For this review, take the finished solid that the model builds, in its own axes (mm). A direction names the side the tool comes from. Round coordinates to 2 decimals unless told otherwise and drop trailing zeros. Loops run counter-clockwise (first coordinate to the right, second up) from the corner with the lowest first, then second, coordinate; pieces in that order, holes last. Notation, with made-up numbers: (-31, -15.75) -> (-13, -15.75) arc R35 ccw to (-13, 16.25) -> close; hole circle Ø2 at (57, 31). An arc over 180 degrees is marked (long way). Write each question's results on one line, items separated by ' | '.
```python
from build123d import *

# Parameters (mm, degrees)
SKETCH2_W               = 300
SKETCH2_H               = 292.795139568
SKETCH2_H_2             = 222.204860432
SKETCH2_H_3             = 20
BOSS_EXTRUDE1_DEPTH     = 20
SHELL1_T                = -1
SKETCH3_W               = 2
SKETCH3_H               = 20
BOSS_EXTRUDE2_DEPTH     = 40
CUT_EXTRUDE1_DEPTH      = 960.966652524
CUT_EXTRUDE1_DEPTH_BACK = 960.966652524
SKETCH4_R               = 3.5
CUT_EXTRUDE2_DEPTH      = 847.070903624
CUT_EXTRUDE2_DEPTH_BACK = 847.070903624
SKETCH5_R               = 3.5


with BuildPart() as part:
    # Sketch2 → Boss-Extrude1 (new body)
    with BuildSketch(Plane.XY):
        Polygon((-19.075846715, -602.110166283), (-189.075846715, -602.110166283), (-189.075846715, -627.110166283), (500.924153285, -627.110166283), (500.924153285, -602.110166283), (330.924153285, -602.110166283), (330.924153285, -2.110166283), (-19.075846715, -2.110166283), align=None)
        with Locations((155.924153285, -173.507736067)):
            Rectangle(SKETCH2_W, SKETCH2_H, mode=Mode.SUBTRACT)
        with Locations((155.924153285, -491.007736067)):
            Rectangle(SKETCH2_W, SKETCH2_H_2, mode=Mode.SUBTRACT)
        with Locations((155.924153285, -349.905305851)):
            Rectangle(SKETCH2_W, SKETCH2_H_3, mode=Mode.SUBTRACT)
    extrude(amount=BOSS_EXTRUDE1_DEPTH)

    # Shell1
    shell1_openings = [part.faces().sort_by_distance(p)[0] for p in [
        (500.924153285, -614.610166283, 10),
        (-189.075846715, -614.610166283, 10),
    ]]
    offset(amount=SHELL1_T, openings=shell1_openings, kind=Kind.INTERSECTION)

    # Sketch3 → Boss-Extrude2 (add)
    with BuildSketch(Plane.XZ.offset(627.110166283)):
        with Locations((493.924153285, 10)):
            Rectangle(SKETCH3_W, SKETCH3_H)
        with Locations((-182.075846715, 10)):
            Rectangle(SKETCH3_W, SKETCH3_H)
    extrude(amount=BOSS_EXTRUDE2_DEPTH)

    # Sketch4 → Cut-Extrude1 (cut, two sides: drawn at the far end of the back side and taken through both)
    with BuildSketch(Plane.ZY.offset(189.075846715).offset(-CUT_EXTRUDE1_DEPTH_BACK)):
        with Locations((10, -652.110166283)):
            Circle(SKETCH4_R)
    extrude(amount=CUT_EXTRUDE1_DEPTH + CUT_EXTRUDE1_DEPTH_BACK, mode=Mode.SUBTRACT)

    # Sketch5 → Cut-Extrude2 (cut, two sides: drawn at the far end of the back side and taken through both)
    with BuildSketch(Plane.ZY.offset(19.075846715).offset(-CUT_EXTRUDE2_DEPTH_BACK)):
        with Locations(Location((10, -273.200166283, 0), (0, 0, 270))):
            Circle(SKETCH5_R)
    extrude(amount=CUT_EXTRUDE2_DEPTH + CUT_EXTRUDE2_DEPTH_BACK, mode=Mode.SUBTRACT)


solid = part.part
```
1. Consider section A-A (x = 177.5). Give the number of separate pieces and of enclosed holes in the cut face, plus the area to 3 significant figures.
Values found:
separate pieces: 4 | enclosed holes: 4 | area: 324 mm2
2. Consider section C-C (y = -613.5). State the section outline as (x, z) points, plus the area to 3 significant figures.
Values found:
outline: (-189.08, 0) -> (500.92, 0) -> (500.92, 1) -> (-189.08, 1) -> close; (-189.08, 19) -> (500.92, 19) -> (500.92, 20) -> (-189.08, 20) -> close | area: 1,380 mm2
3. Tool access review of faces 4 (the face through (154, -602.11, 10)), 5 (the face through (492.924, -647, 10)), 6 (the face through (306.924, -176, 10)): name each direction out of +Z, -Z, +X, -X, +Y, -Y from which nothing blocks a thin tool from reaching the whole face with its end or side.
Values found:
face 4: +Z, -Z | face 5: +Z, -Z, -Y | face 6: none
4. To check wall thickness, follow probe 1 along X at (y, z) = (-52, 7); probe 2 along Y at (x, z) = (494.3, 10); probe 3 along Y at (x, z) = (5.5, 9.75). State the ranges of each line that lie inside material, in increasing order.
Values found:
probe 1: x = -19.08 to -18.08, 4.92 to 5.92, 305.92 to 306.92, 329.92 to 330.92 | probe 2: y = -667.11 to -655.61, -648.61 to -626.11, -603.11 to -602.11 | probe 3: y = -627.11 to -626.11, -603.11 to -378.91, -360.91 to -338.91, -320.91 to -276.69, -269.71 to -26.11, -3.11 to -2.11
5. For pin 1 (3 mm diameter, centred on x = -185.5, z = 7.5, fed in from -Y); pin 2 (5 mm diameter, centred on x = 365.5, z = 7.5, fed in from +Y); pin 3 (11 mm diameter, centred on y = -652.11, z = 10, fed in from +X), all flat-tipped, find the tip position at first contact; note any pin that passes through.
Values found:
pin 1: stops at y = -627.11 | pin 2: stops at y = -602.11 | pin 3: stops at x = 494.92
6. Consider section D-D (x = 371). State the section outline as (y, z) points, plus the area to 3 significant figures.
Values found:
outline: (-627.11, 0) -> (-602.11, 0) -> (-602.11, 20) -> (-627.11, 20) -> close; hole (-626.11, 1) -> (-603.11, 1) -> (-603.11, 19) -> (-626.11, 19) -> close | area: 86.0 mm2
7. Draft analysis for pull direction Z (two halves, no side actions). For faces 1 (the face through (154, -333, 0)), 2 (the face through (151, -627.11, 10)), 3 (the face through (306.924, -493, 10)), state which applies: released by +Z, released by -Z, zero draft, split by the parting line, or undercut.
Values found:
face 1: released by -Z | face 2: zero draft | face 3: undercut
8. Consider section B-B (y = -310). State the section outline as (x, z) points, plus the area to 3 significant figures.
Values found:
outline: (-19.08, 0) -> (5.92, 0) -> (5.92, 20) -> (-19.08, 20) -> close; (305.92, 0) -> (330.92, 0) -> (330.92, 20) -> (305.92, 20) -> close; hole (-18.08, 1) -> (4.92, 1) -> (4.92, 19) -> (-18.08, 19) -> close; hole (306.92, 1) -> (329.92, 1) -> (329.92, 19) -> (306.92, 19) -> close | area: 172 mm2
